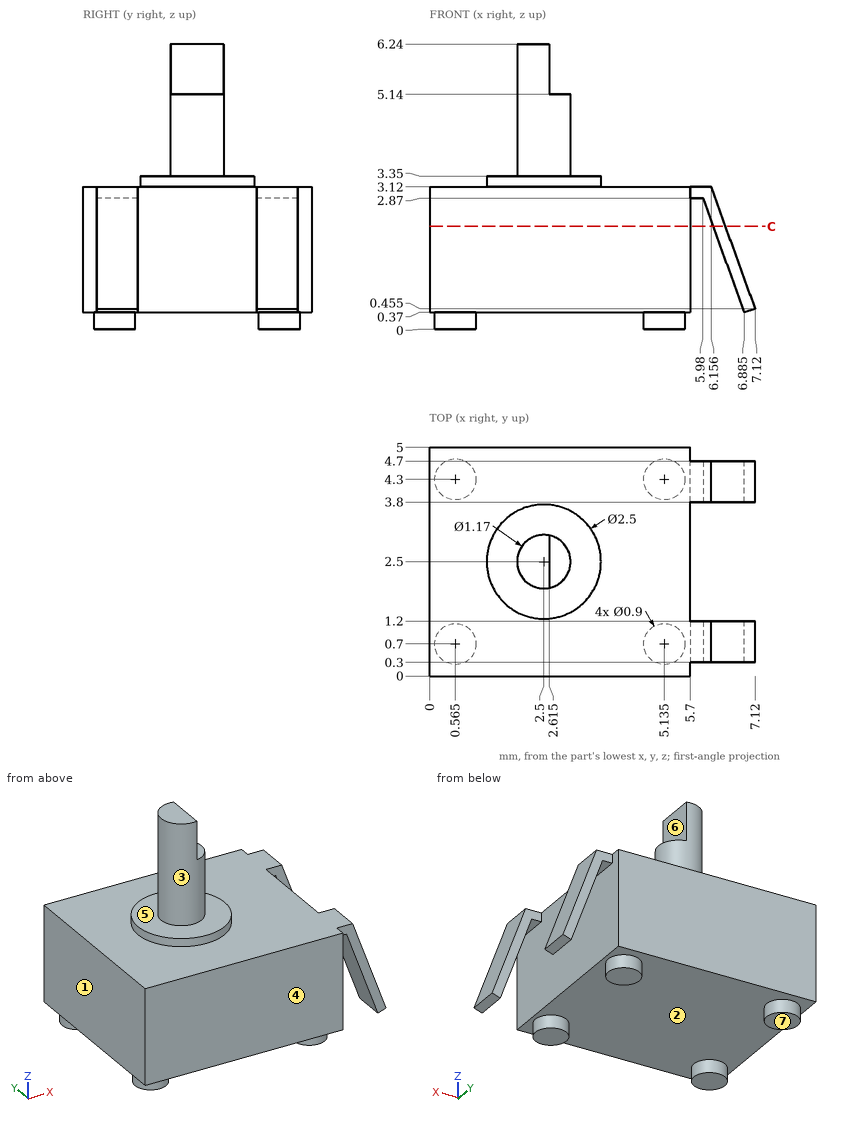
Answer from the drawing. Dimensions are ordinates in mm from the lowest x, y and z of the part. A direction names the side the tool comes from. Give positions to 0.01 mm unless a question says otherwise; leave off trailing zeros.
(1) For the marked faces 5, 6 and 7, determine the directions among +Z, -Z, +X, -X, +Y, -Y from which every point of the face is accessible in a straight line to the end or side of a thin tool.
(2) Find section C-C (z = 2.25). Give the number of separate pieces and of enclosed holes in the cut face, plus the area to 3 significant figures.
(3) Given pin 1 (0.7 mm diameter, centred on x = 6.5, z = 1.5, fed in from +Y); pin 2 (0.5 mm diameter, centred on x = 3, y = 2.5, fed in from +Z); pin 3 (3 mm diameter, centred on y = 3.5, z = 2.5, fed in from +X), each flat-ended and moving along its own axis, determine where each tip first touches the part or whether it passes through.
(4) Straight lines are drawn through the part: L1, parallel to Z at x = 0.75, y = 0.35; L2, parallel to Z at x = 1.5, y = 3.9; L3, parallel to X at y = 1.55, z = 3. For each, find the intervals that lie inside material, in ascending order.
(5) For a pull along Y with two mould halves and no side action, classify the marked faces 1, 2, 3 and 4 as released by +Y, released by -Y, zero draft, split by the parting line, or undercut.
Result sheet:
1. face 5: +Z
1. face 6: +Z, +X, +Y, -Y
1. face 7: -Z, +X, -X, +Y, -Y
2. separate pieces: 3
2. enclosed holes: 0
2. area: 29.0 mm2
3. pin 1: stops at y = 4.7
3. pin 2: stops at z = 5.14
3. pin 3: stops at x = 6.91
4. L1: z = 0 to 3.12
4. L2: z = 0.37 to 3.12
4. L3: x = 0 to 5.7
5. face 1: zero draft
5. face 2: undercut
5. face 3: split by the parting line
5. face 4: released by -Y
